Geometry check sheet. Reference: the model listing, model coordinates, mm. A direction names the side the tool comes from. Round coordinates to 2 decimals unless told otherwise and drop trailing zeros. Write each loop counter-clockwise with the first axis right and the second up, starting at its lowest first coordinate (ties: lowest second). Pieces come first, ordered by that corner, then holes.
from build123d import *

# Parameters (mm, degrees)
F0_W     = 37.13936
F0_H     = 1.666666
F1_DEPTH = 30
F2_W     = 37.571562
F2_H     = 20
F3_DEPTH = 3
F4_W     = 37.139
F4_H     = 10
F5_DEPTH = 6


with BuildPart() as f1:
    # F0 (on Front) → F1 (new body)
    with BuildSketch(Plane.XZ):
        with Locations((2.85544, 0)):
            Rectangle(F0_W, F0_H)
    extrude(amount=F1_DEPTH)

    # F2 (on Top) → F3 (join)
    with BuildSketch(Plane.XY):
        with Locations((2.705152, -10)):
            Rectangle(F2_W, F2_H)
    extrude(amount=F3_DEPTH)

    # F4 (on Top) → F5 (join)
    with BuildSketch(Plane.XY):
        with Locations((2.344745, -5)):
            Rectangle(F4_W, F4_H)
    extrude(amount=F5_DEPTH)


solid = f1.part
1. Section check C-C (z = 2.5). Record the cut outline in (x, y).
2. Section check B-B (y = -13). Record the cut outline in (x, z).
3. Section check A-A (x = 18). Record the cut outline in (y, z).
4. Section check D-D (y = -26). Record the cut outline in (x, z).
5. Depth check by flat-ended pin: pin 1 Ø3 at (x, z) = (3.5, 4) entering from -Y; pin 2 Ø8 at (x, y) = (1, -23.5) entering from +Z; pin 3 Ø2.5 at (y, z) = (-7, 4.5) entering from +X; pin 4 Ø1.5 at (x, z) = (6, 4.5) entering from +Y. Enter the tip coordinate at first touch or a pass-through.
6. Access from +Z, -Z, +X, -X, +Y, -Y to the whole of each face (thin tool, end or side, straight path). Record for faces 1 (the face through (3, -25, 0.833)), 2 (the face through (-16.081, -15, 1)), 3 (the face through (20.914, -5, 4)), 4 (the face through (3, -30, 0)).
7. Scan lines: line 1 along Z through (x, y) = (12, -10.25); line 2 along X through (y, z) = (-2.5, 5); line 3 along Y through (x, z) = (-12, 4.25). Record each from-to range of solid material in increasing order.
Results below:
1. outline: (-16.22, -10) - (-16.08, -10) - (-16.08, -20) - (21.49, -20) - (21.49, 0) - (-16.22, 0) - close
2. outline: (-16.08, 0) - (-15.71, 0) - (-15.71, -0.83) - (21.43, -0.83) - (21.43, 0) - (21.49, 0) - (21.49, 3) - (-16.08, 3) - close
3. outline: (-30, -0.83) - (0, -0.83) - (0, 6) - (-10, 6) - (-10, 3) - (-20, 3) - (-20, 0.83) - (-30, 0.83) - close
4. outline: (-15.71, -0.83) - (21.43, -0.83) - (21.43, 0.83) - (-15.71, 0.83) - close
5. pin 1: stops at y = -20
5. pin 2: stops at z = 3
5. pin 3: stops at x = 20.91
5. pin 4: stops at y = 0
6. face 1: +Z, +X, -X, -Y
6. face 2: +Z, -Z, -X, -Y
6. face 3: +Z, +X, +Y, -Y
6. face 4: +Z, -Z, +X, -X, -Y
7. line 1: z = -0.83 to 3
7. line 2: x = -16.22 to 20.91
7. line 3: y = -10 to 0
